Geometry: final body of the model. Coordinates: model frame, mm. A direction names the side the tool comes from. Give positions to 0.01 mm unless a question says otherwise; leave off trailing zeros. Write each loop counter-clockwise with the first axis right and the second up, starting at its lowest first coordinate (ties: lowest second). Pieces come first, ordered by that corner, then holes. Notation, with made-up numbers: (-19.5, 30) -> (-0.5, 30) arc R28 ccw to (-0.5, 53) -> close; hole circle Ø6 at (23, 52.5). An arc over 180 degrees is marked (long way). Answer as a JSON object with one key per item and string values. Group by question number.
(1) Draft query along X for faces 3 (the face through (-32.825, -52.464, 1.521)), 4 (the face through (-25, -53, 1)), 5 (the face through (-12, -27, 0)). Return one class per face: +X half, -X half, draft (parallel to the pull), parting line (faces both ways), or undercut.
(2) Contact query for flat-ended pins moving along their axis: pin 1 Ø2.5 at (x, y) = (-2, -7.5) entering from +Z; pin 2 Ø1.5 at (x, z) = (12.5, 2) entering from -Y. Output: stop coordinate, or through.
(3) Set-up query: faces 1 (the face through (-20, -20, 1)), 2 (the face through (13, -15, 1)). Return all of +Z, -Z, +X, -X, +Y, -Y with unobstructed straight access to the full face (end or side cutting, diameter ignored); none if empty.
(4) Section query D-D on x = -32.5. Output: boundary loops of the cut face in (y, z).
(5) Material intervals for probe 1 along Y at (x, z) = (-32.5, 1.9); probe 2 along Y at (x, z) = (-2, 2.35); probe 3 along X at (y, z) = (-38.5, 0.2), sorted ascending.
(6) Section query A-A on x = -2. Output: boundary loops of the cut face in (y, z), plus the area to 3 significant figures.
(7) Section query C-C on y = -38. Output: boundary loops of the cut face in (x, z), plus the area to 3 significant figures.
(8) Section query B-B on y = -7.5. Output: boundary loops of the cut face in (x, z), plus the area to 3 significant figures.
from build123d import *

# Parameters (mm, degrees)
EXTRUDE_1_DEPTH     = 3
SKETCH_2_R          = 1.5
CUT_EXTRUDE_1_DEPTH = 3


with BuildPart() as part:
    # 草图1 → 凸台-拉伸1 (new body)
    with BuildSketch(Plane.XY):
        with BuildLine():
            Line((0, 0), (15, 0))
            Line((15, 0), (15, -15))
            Line((15, -15), (11.142135624, -15))
            ThreePointArc((11.142135624, -15), (7.3153013, -15.761204675), (4.071067812, -17.928932188))
            Line((4.071067812, -17.928932188), (-22.071067812, -44.071067812))
            ThreePointArc((-22.071067812, -44.071067812), (-24.238795325, -47.3153013), (-25, -51.142135624))
            Line((-25, -51.142135624), (-25, -55))
            Line((-25, -55), (-40, -55))
            Line((-40, -55), (-40, -40))
            Line((-40, -40), (0, 0))
        make_face()
    extrude(amount=EXTRUDE_1_DEPTH)

    # 草图2 → 切除-拉伸1 (cut)
    with BuildSketch(Plane.XY.offset(3)):
        with Locations((11, -7.5)):
            Circle(SKETCH_2_R)
        with Locations((-2, -7.5)):
            Circle(SKETCH_2_R)
        with Locations((-32.5, -51)):
            Circle(SKETCH_2_R)
        with Locations((-32.5, -38)):
            Circle(SKETCH_2_R)
    extrude(amount=-CUT_EXTRUDE_1_DEPTH, mode=Mode.SUBTRACT)


solid = part.part
Answer list:
{
 "1": {"face 3": "undercut", "face 4": "+X half", "face 5": "draft"},
 "2": {"pin 1": "through", "pin 2": "y = -15"},
 "3": {"face 1": "+Z, -Z, -X, +Y", "face 2": "+Z, -Z, +X, -Y"},
 "4": {"outline": "(-55, 0) -> (-52.5, 0) -> (-52.5, 3) -> (-55, 3) -> close; (-49.5, 0) -> (-39.5, 0) -> (-39.5, 3) -> (-49.5, 3) -> close; (-36.5, 0) -> (-32.5, 0) -> (-32.5, 3) -> (-36.5, 3) -> close"},
 "5": {"probe 1": "-55 to -52.5, -49.5 to -39.5, -36.5 to -32.5", "probe 2": "-24 to -9, -6 to -2", "probe 3": "-38.5 to -33.91, -31.09 to -16.5"},
 "6": {"outline": "(-24, 0) -> (-9, 0) -> (-9, 3) -> (-24, 3) -> close; (-6, 0) -> (-2, 0) -> (-2, 3) -> (-6, 3) -> close", "area": "57.0 mm2"},
 "7": {"outline": "(-38, 0) -> (-34, 0) -> (-34, 3) -> (-38, 3) -> close; (-31, 0) -> (-16, 0) -> (-16, 3) -> (-31, 3) -> close", "area": "57.0 mm2"},
 "8": {"outline": "(-7.5, 0) -> (-3.5, 0) -> (-3.5, 3) -> (-7.5, 3) -> close; (-0.5, 0) -> (9.5, 0) -> (9.5, 3) -> (-0.5, 3) -> close; (12.5, 0) -> (15, 0) -> (15, 3) -> (12.5, 3) -> close", "area": "49.5 mm2"}
}
